Input: part model. Units: mm. Frame: model coordinates. A direction names the side the tool comes from. Round coordinates to 2 decimals unless told otherwise and drop trailing zeros. Loops run counter-clockwise (first coordinate to the right, second up) from the corner with the lowest first, then second, coordinate; pieces in that order, holes last. Notation, with made-up numbers: (16, -31) -> (36, -31) arc R6 cw to (36, -25) -> close; hole circle Ø5 at (49.5, -26). An arc over 180 degrees is marked (long way). Answer in a Markdown table with one row per item. Add a question column.
Q1. Section C-C, the plane y = 26. Output: boundary loops of the cut face in (x, z).
Q2. Section B-B, the plane x = -9. Output: boundary loops of the cut face in (y, z).
Q3. Section A-A, the plane y = 21.5. Output: boundary loops of the cut face in (x, z).
Q4. Mould query, pull axis X, two halves, no side actions, for faces 1 (the face through (14.1, 1.6, -25.7)), 2 (the face through (0, 3, 34)), 3 (the face through (29.1, 11, 0)). Classes: pulls with the +X half, pulls with the -X half, needs draft (parallel to the pull), parting line crosses it, or undercut.
Q5. Section D-D, the plane y = 3. Output: boundary loops of the cut face in (x, z).
Q6. Ray query, L1, parallel to Y at x = 29, z = 0; L2, parallel to Y at x = 31.25, z = 0; L3, parallel to X at y = 24, z = 10. Return the intervals inside material, ascending. Write a range as from..to.
Q7. Pin query (flat end, axial travel): pin 1 (10 mm diameter, centred on x = 18.5, z = -14, fed in from +Y); pin 2 (15 mm diameter, centred on x = -23, y = 17.5, fed in from +Z); pin 3 (1.5 mm diameter, centred on y = 17, z = -4, fed in from -X). Return the tip coordinate at first contact, or that it passes through.
Q8. Reachability of faces 4 (the face through (25.5, 30, -3)), 5 (the face through (-24.13, 25.12, -1.08)), 6 (the face through (30, 18, -12.5)) from +Z, -Z, +X, -X, +Y, -Y: full face, straight path, thin tool, end or side. Return the list, or none.
```python
from build123d import *

# Parameters (mm, degrees)
BOSS_EXTRUDE1_DEPTH  = 2
SKETCH2_W            = 28.2
SKETCH2_H            = 9.8
BOSS_EXTRUDE2_DEPTH  = 2
FILLET1_R            = 4
FILLET1_OF_MIRROR2_R = 4
SKETCH3_W            = 25
SKETCH3_H            = 40
SKETCH3_R            = 2.5
BOSS_EXTRUDE3_DEPTH  = 7.6
FILLET2_R            = 4
CUT_EXTRUDE1_REACH   = 71.698
SKETCH4_W            = 3.6
SKETCH4_H            = 18
SKETCH5_R            = 5
BOSS_EXTRUDE4_DEPTH  = 4


with BuildPart() as part:
    # Sketch1 → Boss-Extrude1 (new body)
    with BuildSketch(Plane(origin=(0, 0, 0), x_dir=(1, 0, 0), z_dir=(0, 1, 0))):
        Polygon((-14.1, 12.5), (-14.1, 34), (14.1, 34), (14.1, 12.5), (33.1, 12.5), (33.1, -12.5), (14.1, -12.5), (14.1, -34), (-14.1, -34), (-14.1, -12.5), (-33.1, -12.5), (-33.1, 12.5), align=None)
    boss_extrude1 = extrude(amount=BOSS_EXTRUDE1_DEPTH)

    # Sketch2 → Boss-Extrude2 (add)
    with BuildSketch(Plane.XY.offset(34)):
        with Locations((0, 4.9)):
            Rectangle(SKETCH2_W, SKETCH2_H)
    boss_extrude2 = extrude(amount=-BOSS_EXTRUDE2_DEPTH)

    # Fillet1
    # the kernel refuses this fillet: 4 mm, written as the material it takes off along each edge
    with BuildSketch(Plane(origin=(-22.760254038, 9.8, 34), x_dir=(0, -1, 0), z_dir=(1, 0, 0))) as fillet1_piece_1:
        with BuildLine():
            CenterArc((3.464101615, 4), FILLET1_R, 210, 60)
            Line((0, 2), (-0.069282032, 1.96))
            ThreePointArc((-0.069282032, 1.96), (-0.08, 1), (-0.08, 0))
            Line((-0.08, 0), (0, -0.08))
            Line((0, -0.08), (3.464101615, -0.08))
            Line((3.464101615, -0.08), (3.464101615, 0))
        make_face()
    extrude(amount=45.520508076, mode=Mode.SUBTRACT)

    # Mirror2: Boss-Extrude1, Boss-Extrude2 across plane
    add(boss_extrude1.mirror(Plane.XY))
    add(boss_extrude2.mirror(Plane.XY))

    # Fillet1 of Mirror2
    # the kernel refuses this fillet: 4 mm, written as the material it takes off along each edge
    with BuildSketch(Plane(origin=(-22.760254038, 9.8, -34), x_dir=(0, -1, 0), z_dir=(1, 0, 0))) as fillet1_of_mirror2_piece_1:
        with BuildLine():
            CenterArc((3.464101615, -4), FILLET1_OF_MIRROR2_R, 90, 60)
            Line((0, -2), (-0.069282032, -1.96))
            ThreePointArc((-0.069282032, -1.96), (-0.08, -1), (-0.08, 0))
            Line((-0.08, 0), (0, 0.08))
            Line((0, 0.08), (3.464101615, 0.08))
            Line((3.464101615, 0.08), (3.464101615, 0))
        make_face()
    extrude(amount=45.520508076, mode=Mode.SUBTRACT)

    # Sketch3 → Boss-Extrude3 (add)
    with BuildSketch(Plane(origin=(33.1, 0, 0), x_dir=(0, 0, -1), z_dir=(1, 0, 0))):
        with Locations((0, 20)):
            Rectangle(SKETCH3_W, SKETCH3_H)
        with Locations((0, 30)):
            Circle(SKETCH3_R, mode=Mode.SUBTRACT)
    extrude(amount=-BOSS_EXTRUDE3_DEPTH)

    # Fillet2
    fillet2_edges = [part.edges().sort_by_distance(p)[0] for p in [
        (29.3, 40, -12.5),
        (29.3, 40, 12.5),
    ]]
    fillet(fillet2_edges, radius=FILLET2_R)

    # Sketch4 → Cut-Extrude1 (cut, up to next)
    with BuildSketch(Plane.XY.offset(12.5), mode=Mode.PRIVATE) as cut_extrude1_sk1:
        with Locations((27.3, 11)):
            Rectangle(SKETCH4_W, SKETCH4_H)
    cut_extrude1_tool1 = extrude(cut_extrude1_sk1.sketch, amount=-CUT_EXTRUDE1_REACH, mode=Mode.PRIVATE) & part.part
    add(cut_extrude1_tool1.solids().sort_by_distance((27.3, 11, 12.5))[0], mode=Mode.SUBTRACT)

    # Sketch5 → Boss-Extrude4 (add)
    with BuildSketch(Plane.ZY.offset(26.1)):
        with BuildLine():
            Line((12.5, 0), (-12.5, 0))
            Line((-12.5, 0), (-12.5, 27.51))
            ThreePointArc((-12.5, 27.51), (-8.841763697, 36.341763697), (-0.01, 40))
            Line((-0.01, 40), (0.01, 40))
            ThreePointArc((0.01, 40), (8.841763697, 36.341763697), (12.5, 27.51))
            Line((12.5, 27.51), (12.5, 0))
        make_face()
        with Locations((0, 30)):
            Circle(SKETCH5_R, mode=Mode.SUBTRACT)
    extrude(amount=-BOSS_EXTRUDE4_DEPTH)


solid = part.part
```
Answer block:
| question | item | result |
|---|---|---|
| 1 | outline | (-26.1, -12.5) -> (-22.1, -12.5) -> (-22.1, -3) -> (-26.1, -3) -> close; (-26.1, 3) -> (-22.1, 3) -> (-22.1, 12.5) -> (-26.1, 12.5) -> close; (25.5, -12.5) -> (33.1, -12.5) -> (33.1, 12.5) -> (25.5, 12.5) -> close |
| 2 | outline | (0, -34) -> (6.34, -34) arc R4 ccw to (9.8, -32) -> (2, -32) -> (2, 32) -> (9.8, 32) arc R4 ccw to (6.34, 34) -> (0, 34) -> close |
| 3 | outline | (-26.1, -12.5) -> (-22.1, -12.5) -> (-22.1, 12.5) -> (-26.1, 12.5) -> close; (25.5, -12.5) -> (33.1, -12.5) -> (33.1, 12.5) -> (25.5, 12.5) -> close |
| 4 | face 1 | pulls with the +X half |
| 4 | face 2 | needs draft |
| 4 | face 3 | undercut |
| 5 | outline | (-26.1, -12.5) -> (-22.1, -12.5) -> (-22.1, 12.5) -> (-26.1, 12.5) -> close; (-14.1, -34) -> (14.1, -34) -> (14.1, -32) -> (-14.1, -32) -> close; (-14.1, 32) -> (14.1, 32) -> (14.1, 34) -> (-14.1, 34) -> close; (29.1, -12.5) -> (33.1, -12.5) -> (33.1, 12.5) -> (29.1, 12.5) -> close |
| 6 | L1 | 0..2, 20..27.5, 32.5..40 |
| 6 | L2 | 0..27.5, 32.5..40 |
| 6 | L3 | -26.1..-22.1, 25.5..33.1 |
| 7 | pin 1 | y = 2 |
| 7 | pin 2 | z = 12.5 |
| 7 | pin 3 | x = -26.1 |
| 8 | face 4 | +Z, -Z, +Y |
| 8 | face 5 | -X |
| 8 | face 6 | -Z, +X, +Y, -Y |
